from build123d import *

# Parameters (mm, degrees)
BASE_FLANGE1_DEPTH = 1613
FILLET1_R          = 3
CUT_EXTRUDE1_REACH = 1625.966
SKETCH6_R          = 11
LPATTERN1_COUNT    = 15
LPATTERN1_PITCH    = 132
CUT_EXTRUDE4_REACH = 1634.045
SKETCH10_R         = 3.25
LPATTERN5_COUNT    = 4
LPATTERN5_PITCH    = 529
CUT_EXTRUDE5_REACH = 1623.619
CUT_EXTRUDE6_REACH = 1623.619
SKETCH13_R         = 3.25
CUT_EXTRUDE7_REACH = 1623.619
SKETCH14_R         = 3.25
LPATTERN6_COUNT    = 3
LPATTERN6_PITCH    = 529
CUT_EXTRUDE8_REACH = 1623.619
SKETCH15_R         = 3.25


# Sheet-metal steps are written as plain solids
with BuildPart() as part:
    # Sketch1 → Base-Flange1 (new body)
    with BuildSketch(Plane(origin=(0, 0, 0), x_dir=(1, 0, 0), z_dir=(0, 1, 0))):
        with BuildLine():
            Line((-113, 149), (-113, 123))
            ThreePointArc((-113, 123), (-112.707106781, 122.292893219), (-112, 122))
            Line((-112, 122), (-61.506905499, 122))
            ThreePointArc((-61.506905499, 122), (-60.303378662, 121.597348789), (-59.584453364, 120.551523153))
            Line((-59.584453364, 120.551523153), (-25.207773318, 0.724238423))
            ThreePointArc((-25.207773318, 0.724238423), (-24.848310669, 0.201325606), (-24.246547251, 0))
            Line((-24.246547251, 0), (24.246547251, 0))
            ThreePointArc((24.246547251, 0), (24.848310669, 0.201325606), (25.207773318, 0.724238423))
            Line((25.207773318, 0.724238423), (59.584453364, 120.551523153))
            ThreePointArc((59.584453364, 120.551523153), (60.303378662, 121.597348789), (61.506905499, 122))
            Line((61.506905499, 122), (87, 122))
            ThreePointArc((87, 122), (87.707106781, 122.292893219), (88, 123))
            Line((88, 123), (88, 149))
            Line((88, 149), (89, 149))
            Line((89, 149), (89, 123))
            ThreePointArc((89, 123), (88.414213562, 121.585786438), (87, 121))
            Line((87, 121), (61.506905499, 121))
            ThreePointArc((61.506905499, 121), (60.90514208, 120.798674394), (60.545679431, 120.275761577))
            Line((60.545679431, 120.275761577), (26.168999386, 0.448476847))
            ThreePointArc((26.168999386, 0.448476847), (25.450074087, -0.597348789), (24.246547251, -1))
            Line((24.246547251, -1), (-24.246547251, -1))
            ThreePointArc((-24.246547251, -1), (-25.450074087, -0.597348789), (-26.168999386, 0.448476847))
            Line((-26.168999386, 0.448476847), (-60.545679431, 120.275761577))
            ThreePointArc((-60.545679431, 120.275761577), (-60.90514208, 120.798674394), (-61.506905499, 121))
            Line((-61.506905499, 121), (-112, 121))
            ThreePointArc((-112, 121), (-113.414213562, 121.585786438), (-114, 123))
            Line((-114, 123), (-114, 149))
            Line((-114, 149), (-113, 149))
        make_face()
    extrude(amount=BASE_FLANGE1_DEPTH)

    # Fillet1
    fillet1_edges = [part.edges().sort_by_distance(p)[0] for p in [
        (-113.5, 0, -149),
        (88.5, 0, -149),
        (-113.5, 1613, -149),
        (88.5, 1613, -149),
    ]]
    fillet(fillet1_edges, radius=FILLET1_R)

    # Sketch6 → Cut-Extrude1 (cut, up to next)
    with BuildSketch(Plane.XY.offset(1), mode=Mode.PRIVATE) as cut_extrude1_sk1:
        with Locations((0, 79)):
            Circle(SKETCH6_R)
    cut_extrude1_tool1 = extrude(cut_extrude1_sk1.sketch, amount=-CUT_EXTRUDE1_REACH, mode=Mode.PRIVATE) & part.part
    cut_extrude1 = cut_extrude1_tool1.solids().sort_by_distance((0, 79, 1))[0]
    add(cut_extrude1, mode=Mode.SUBTRACT)

    # LPattern1: Cut-Extrude1 ×15
    with Locations(*[(0, i * LPATTERN1_PITCH, 0) for i in range(1, LPATTERN1_COUNT)]):
        add(cut_extrude1, mode=Mode.SUBTRACT)

    # Cut-Extrude4: up to this face of the body (flat: up to its plane)
    cut_extrude4_end = Plane(part.part.faces().sort_by_distance((-114, 806.5, -135.998864211))[0])
    # Sketch10 → Cut-Extrude4 (cut, up to the picked face)
    with BuildSketch(Plane(origin=(89, 0, -5.5), x_dir=(0, 0, -1), z_dir=(1, 0, 0)), mode=Mode.PRIVATE) as cut_extrude4_sk1:
        with Locations((133.5, 13)):
            Circle(SKETCH10_R)
    cut_extrude4_tool1 = split(extrude(cut_extrude4_sk1.sketch, amount=-CUT_EXTRUDE4_REACH, mode=Mode.PRIVATE), bisect_by=cut_extrude4_end, keep=Keep.BOTH, mode=Mode.PRIVATE)
    cut_extrude4 = cut_extrude4_tool1.solids().sort_by(Axis((89, 13, -139), (-1, 0, 0)))[0]
    add(cut_extrude4, mode=Mode.SUBTRACT)

    # LPattern5: Cut-Extrude4 ×4
    with Locations(*[(0, i * LPATTERN5_PITCH, 0) for i in range(1, LPATTERN5_COUNT)]):
        add(cut_extrude4, mode=Mode.SUBTRACT)

    # Sketch12 → Cut-Extrude5 (cut, up to next)
    with BuildSketch(Plane.XY.offset(-121), mode=Mode.PRIVATE) as cut_extrude5_sk1:
        with BuildLine():
            Line((-100.006905499, 99.5), (-100.006905499, 124.5))
            ThreePointArc((-100.006905499, 124.5), (-85.006905499, 139.5), (-70.006905499, 124.5))
            Line((-70.006905499, 124.5), (-70.006905499, 99.5))
            ThreePointArc((-70.006905499, 99.5), (-85.006905499, 84.5), (-100.006905499, 99.5))
        make_face()
    cut_extrude5_tool1 = extrude(cut_extrude5_sk1.sketch, amount=-CUT_EXTRUDE5_REACH, mode=Mode.PRIVATE) & part.part
    # Sketch12 → Cut-Extrude5 (cut, up to next)
    with BuildSketch(Plane.XY.offset(-121), mode=Mode.PRIVATE) as cut_extrude5_sk2:
        with BuildLine():
            Line((-100.006905499, 1187.5), (-100.006905499, 1212.5))
            ThreePointArc((-100.006905499, 1212.5), (-85.006905499, 1227.5), (-70.006905499, 1212.5))
            Line((-70.006905499, 1212.5), (-70.006905499, 1187.5))
            ThreePointArc((-70.006905499, 1187.5), (-85.006905499, 1172.5), (-100.006905499, 1187.5))
        make_face()
    cut_extrude5_tool2 = extrude(cut_extrude5_sk2.sketch, amount=-CUT_EXTRUDE5_REACH, mode=Mode.PRIVATE) & part.part
    # Sketch12 → Cut-Extrude5 (cut, up to next)
    with BuildSketch(Plane.XY.offset(-121), mode=Mode.PRIVATE) as cut_extrude5_sk3:
        with BuildLine():
            Line((-70.006905499, 1512.5), (-70.006905499, 1487.5))
            ThreePointArc((-70.006905499, 1487.5), (-85.006905499, 1472.5), (-100.006905499, 1487.5))
            Line((-100.006905499, 1487.5), (-100.006905499, 1512.5))
            ThreePointArc((-100.006905499, 1512.5), (-85.006905499, 1527.5), (-70.006905499, 1512.5))
        make_face()
    cut_extrude5_tool3 = extrude(cut_extrude5_sk3.sketch, amount=-CUT_EXTRUDE5_REACH, mode=Mode.PRIVATE) & part.part
    add(cut_extrude5_tool1.solids().sort_by_distance((-85.006905, 112, -121))[0], mode=Mode.SUBTRACT)
    add(cut_extrude5_tool2.solids().sort_by_distance((-85.006905, 1200, -121))[0], mode=Mode.SUBTRACT)
    add(cut_extrude5_tool3.solids().sort_by_distance((-85.006905, 1500, -121))[0], mode=Mode.SUBTRACT)

    # Sketch13 → Cut-Extrude6 (cut, up to next)
    with BuildSketch(Plane.XY.offset(-121), mode=Mode.PRIVATE) as cut_extrude6_sk1:
        with Locations((-86.506905499, 25)):
            Circle(SKETCH13_R)
    cut_extrude6_tool1 = extrude(cut_extrude6_sk1.sketch, amount=-CUT_EXTRUDE6_REACH, mode=Mode.PRIVATE) & part.part
    cut_extrude6 = cut_extrude6_tool1.solids().sort_by_distance((-86.506905, 25, -121))[0]
    add(cut_extrude6, mode=Mode.SUBTRACT)

    # Sketch14 → Cut-Extrude7 (cut, up to next)
    with BuildSketch(Plane.XY.offset(-121), mode=Mode.PRIVATE) as cut_extrude7_sk1:
        with Locations((74.006905499, 25)):
            Circle(SKETCH14_R)
    cut_extrude7_tool1 = extrude(cut_extrude7_sk1.sketch, amount=-CUT_EXTRUDE7_REACH, mode=Mode.PRIVATE) & part.part
    cut_extrude7 = cut_extrude7_tool1.solids().sort_by_distance((74.006905, 25, -121))[0]
    add(cut_extrude7, mode=Mode.SUBTRACT)

    # LPattern6: Cut-Extrude6, Cut-Extrude7 ×3
    with Locations(*[(0, i * LPATTERN6_PITCH, 0) for i in range(1, LPATTERN6_COUNT)]):
        add(cut_extrude6, mode=Mode.SUBTRACT)
        add(cut_extrude7, mode=Mode.SUBTRACT)

    # Sketch15 → Cut-Extrude8 (cut, up to next)
    with BuildSketch(Plane.XY.offset(-121), mode=Mode.PRIVATE) as cut_extrude8_sk1:
        with Locations((-86.506905499, 1588)):
            Circle(SKETCH15_R)
    cut_extrude8_tool1 = extrude(cut_extrude8_sk1.sketch, amount=-CUT_EXTRUDE8_REACH, mode=Mode.PRIVATE) & part.part
    # Sketch15 → Cut-Extrude8 (cut, up to next)
    with BuildSketch(Plane.XY.offset(-121), mode=Mode.PRIVATE) as cut_extrude8_sk2:
        with Locations((74.006905499, 1588)):
            Circle(SKETCH15_R)
    cut_extrude8_tool2 = extrude(cut_extrude8_sk2.sketch, amount=-CUT_EXTRUDE8_REACH, mode=Mode.PRIVATE) & part.part
    add(cut_extrude8_tool1.solids().sort_by_distance((-86.506905, 1588, -121))[0], mode=Mode.SUBTRACT)
    add(cut_extrude8_tool2.solids().sort_by_distance((74.006905, 1588, -121))[0], mode=Mode.SUBTRACT)


solid = part.part
Build history of the part. All positions in model axes, mm. A direction names the side the tool comes from. Coordinates: 2 decimals unless noted, no trailing zeros. Write each loop counter-clockwise with the first axis right and the second up, starting at its lowest first coordinate (ties: lowest second). Pieces come first, ordered by that corner, then holes.
(1) Mould opens along X. For faces 4 (the flat face through (74, 795, -121)), 5 (the flat face through (89, 795, -136)), 6 (the flat face through (74, 795, -122)), 7 (the flat face through (-42.637, 795.209, -61.477)) say: pulls with the +X half, pulls with the -X half, needs draft (parallel to the pull), parting line crosses it, or undercut.
(2) Drill centre lines: line 1 (X direction, y = 211, z = 0.2); line 2 (X direction, y = 1032.5, z = -125); line 3 (Z direction, x = 88.75, y = 1600). Where is each one in solid material? Low to high.
(3) 3-axis set-ups, long thin cutter, end or side, ignore diameter. For faces 1 (the flat face through (43.598, 795.209, -61.201)), 2 (the flat face through (-87, 795, -122)), 3 (the flat face through (-86, 795, -121)): which of +Z, -Z, +X, -X, +Y, -Y reach the whole face in a straight line?
(4) Cut at B-B on y = 390.5. List the corners of the cut face in (x, z).
(5) Cut at A-A on z = -31.5. List the corners of the cut face in (x, y).
(6) Pin check, flat tips, straight feed: pin 1 Ø8 at (y, z) = (210.5, -59.5) entering from -X; pin 2 Ø24 at (x, y) = (-9, 784.5) entering from -Z; pin 3 Ø4 at (y, z) = (13, -139) entering from -X; pin 4 Ø8 at (y, z) = (534.5, -36.5) entering from -X. Stop position of each tip, or through.
Working result:
1. face 4: needs draft
1. face 5: pulls with the +X half
1. face 6: undercut
1. face 7: undercut
2. line 1: x = -25.85 to -11, 11 to 25.85
2. line 2: x = -114 to -113, 88 to 89
2. line 3: z = -149 to -142.25, -135.75 to -122.03
3. face 1: +Z, +X, +Y, -Y
3. face 2: -Z, +Y, -Y
3. face 3: +Z, -X, +Y, -Y
4. outline: (-114, -149) - (-113, -149) - (-113, -123) arc R1 cw to (-112, -122) - (-61.51, -122) arc R2 ccw to (-59.58, -120.55) - (-25.21, -0.72) arc R1 cw to (-24.25, 0) - (24.25, 0) arc R1 cw to (25.21, -0.72) - (59.58, -120.55) arc R2 ccw to (61.51, -122) - (87, -122) arc R1 cw to (88, -123) - (88, -149) - (89, -149) - (89, -123) arc R2 ccw to (87, -121) - (61.51, -121) arc R1 cw to (60.55, -120.28) - (26.17, -0.45) arc R2 ccw to (24.25, 1) - (-24.25, 1) arc R2 ccw to (-26.17, -0.45) - (-60.55, -120.28) arc R1 cw to (-61.51, -121) - (-112, -121) arc R2 ccw to (-114, -123) - close
5. outline: (-35.08, 0) - (-34.04, 0) - (-34.04, 1613) - (-35.08, 1613) - close; (34.04, 0) - (35.08, 0) - (35.08, 1613) - (34.04, 1613) - close
6. pin 1: stops at x = -44.26
6. pin 2: stops at z = 0
6. pin 3: passes through
6. pin 4: stops at x = -37.66
